CAD build for the part. Positions are in the model's coordinates, mm. A direction names the side the tool comes from. Coordinates: 2 decimals unless noted, no trailing zeros. Write each loop counter-clockwise with the first axis right and the second up, starting at its lowest first coordinate (ties: lowest second). Pieces come first, ordered by that corner, then holes. Notation, with made-up numbers: (4, 70) -> (19, 70) arc R20 cw to (19, 86) -> close; hole circle Ø10 at (81, 51). An arc over 180 degrees is marked (long way). Answer as CSV lines item,"result".
```python
from build123d import *

# Parameters (mm, degrees)
ESBO_O1_W                  = 20
ESBO_O1_H                  = 40
RESSALTO_EXTRUS_O1_DEPTH   = 4
ESBO_O2_R                  = 2.3
CORTE_EXTRUS_O1_DEPTH      = 1
CORTE_EXTRUS_O1_DEPTH_BACK = 5
ESBO_O3_W                  = 5.9
ESBO_O3_H                  = 6
ESBO_O3_H_2                = 7
RESSALTO_EXTRUS_O2_DEPTH   = 2
CHANFRO1_SIZE              = 0.5
ESBO_O4_R                  = 5
CORTE_EXTRUS_O2_DEPTH      = 2.5


with BuildPart() as part:
    # Esboço1 → Ressalto-extrusão1 (new body)
    with BuildSketch(Plane(origin=(0, 0, 0), x_dir=(1, 0, 0), z_dir=(0, 1, 0))):
        Rectangle(ESBO_O1_W, ESBO_O1_H)
    extrude(amount=RESSALTO_EXTRUS_O1_DEPTH)

    # Esboço2 → Corte-extrusão1 (cut, two sides)
    with BuildSketch(Plane(origin=(0, 4, 0), x_dir=(1, 0, 0), z_dir=(0, 1, 0))) as corte_extrus_o1_sk:
        with Locations((0, 10)):
            Circle(ESBO_O2_R)
        with Locations((0, -10)):
            Circle(ESBO_O2_R)
    extrude(amount=CORTE_EXTRUS_O1_DEPTH, mode=Mode.SUBTRACT)
    extrude(corte_extrus_o1_sk.sketch, amount=-CORTE_EXTRUS_O1_DEPTH_BACK, mode=Mode.SUBTRACT)

    # Esboço3 → Ressalto-extrusão2 (add)
    with BuildSketch(Plane.XZ):
        with Locations((0, -4)):
            Rectangle(ESBO_O3_W, ESBO_O3_H)
        with Locations((0, -16.5)):
            Rectangle(ESBO_O3_W, ESBO_O3_H_2)
    extrude(amount=RESSALTO_EXTRUS_O2_DEPTH)

    # Chanfro1
    chanfro1_edges = [part.edges().sort_by_distance(p)[0] for p in [
        (-10, 4, 0),
        (0, 4, 20),
        (-2.3, 4, -10),
        (-2.3, 4, 10),
        (10, 4, 0),
        (0, 4, -20),
    ]]
    chamfer(chanfro1_edges, length=CHANFRO1_SIZE)

    # Esboço4 → Corte-extrusão2 (cut)
    with BuildSketch(Plane.XZ):
        with Locations((0, 10)):
            Circle(ESBO_O4_R)
    extrude(amount=-CORTE_EXTRUS_O2_DEPTH, mode=Mode.SUBTRACT)


solid = part.part
```
Item 1: Saw through at B-B on y = -0.5. Give the cut face in (x, z).
Answer below:
outline,"(-2.95, -20) -> (2.95, -20) -> (2.95, -13) -> (-2.95, -13) -> close; (-2.95, -7) -> (2.95, -7) -> (2.95, -1) -> (-2.95, -1) -> close"
Item 2: Saw through at C-C on x = 0. Give the cut face in (y, z), and give its area (3 significant figures).
Answer below:
outline,"(-2, -20) -> (3.5, -20) -> (4, -19.5) -> (4, -12.8) -> (3.5, -12.3) -> (0, -12.3) -> (0, -13) -> (-2, -13) -> close; (-2, -7) -> (0, -7) -> (0, -7.7) -> (3.5, -7.7) -> (4, -7.2) -> (4, 7.2) -> (3.5, 7.7) -> (2.5, 7.7) -> (2.5, 5) -> (0, 5) -> (0, -1) -> (-2, -1) -> close; (0, 15) -> (2.5, 15) -> (2.5, 12.3) -> (3.5, 12.3) -> (4, 12.8) -> (4, 19.5) -> (3.5, 20) -> (0, 20) -> close"
area,"135 mm2"
Item 3: Saw through at A-A on z = 10. Give the cut face in (x, y).
Answer below:
outline,"(-10, 0) -> (-5, 0) -> (-5, 2.5) -> (-2.3, 2.5) -> (-2.3, 3.5) -> (-2.8, 4) -> (-9.5, 4) -> (-10, 3.5) -> close; (2.3, 2.5) -> (5, 2.5) -> (5, 0) -> (10, 0) -> (10, 3.5) -> (9.5, 4) -> (2.8, 4) -> (2.3, 3.5) -> close"
Item 4: Saw through at D-D on z = 3. Give the cut face in (x, y), and give its area (4 significant figures).
Answer below:
outline,"(-10, 0) -> (10, 0) -> (10, 3.5) -> (9.5, 4) -> (-9.5, 4) -> (-10, 3.5) -> close"
area,"79.75 mm2"
Item 5: 3-axis set-ups, long thin cutter, end or side, ignore diameter. For faces 4 (the flat face through (0, -1, -1)), 5 (the flat face through (0, -1, -13)), 6 (the flat face through (2.95, -1, -4)), 7 (the flat face through (2.2, 2.5, 11.2)): which of +Z, -Z, +X, -X, +Y, -Y reach the whole face in a straight line?
Answer below:
face 4,"+Z, +X, -X, -Y"
face 5,"+X, -X, -Y"
face 6,"+Z, -Z, +X, -Y"
face 7,"-Y"
Item 6: Two-plate mould, pull along X, no slides. Class faces 1 (the flat face through (0, 2, 20)), 2 (the cylindrical face through (-0.651, 1.232, 14.957)), 3 (the flat face through (-10, 2, 0)): pulls with the +X half, pulls with the -X half, needs draft (parallel to the pull), parting line crosses it, or undercut.
Answer below:
face 1,"needs draft"
face 2,"undercut"
face 3,"pulls with the -X half"
Item 7: Wall check: line 1 (Z direction, x = 0, y = 2.85); line 2 (Z direction, x = 0, y = 1.1); line 3 (X direction, y = 3.15, z = 10). Give the ranges that are in metal, low to high. Write a range as from..to.
Answer below:
line 1,"z = -20..-12.3, -7.7..7.7, 12.3..20"
line 2,"z = -20..-12.3, -7.7..5, 15..20"
line 3,"x = -10..-2.3, 2.3..10"
Item 8: Flat gauge pins, fed straight in: pin 1 (6 mm diameter, centred on x = 0, z = 6.5, fed in from -Y); pin 2 (0.6 mm diameter, centred on x = -1, y = -0.5, fed in from +Z); pin 3 (0.6 mm diameter, centred on y = -0.5, z = -17, fed in from -X). Where does each tip first touch, or does it go through?
Answer below:
pin 1,"stops at y = 0"
pin 2,"stops at z = -1"
pin 3,"stops at x = -2.95"
